CAD build for the part. Positions are in the model's coordinates, mm. Round coordinates to 2 decimals unless told otherwise and drop trailing zeros. Loops run counter-clockwise (first coordinate to the right, second up) from the corner with the lowest first, then second, coordinate; pieces in that order, holes last.
Autodesk Inventor part; units mm, degrees
ref_plane "YZ Plane" through (0, 0, 0) normal (1, 0, 0) x (0, 1, 0)
ref_plane "XZ Plane" through (0, 0, 0) normal (0, 1, 0) x (-1, 0, 0)
ref_plane "XY Plane" through (0, 0, 0) normal (0, 0, 1) x (1, 0, 0)
sketch "Sketch1" plane through (0, 0, 0) normal (0, 1, 0) x (-1, 0, 0)
  line L0 (0, 0) -> (-298.45, 0)
  line L1 (-298.45, 0) -> (-298.45, 171.45)
  line L2 (-298.45, 171.45) -> (0, 171.45)
  line L3 (0, 171.45) -> (0, 0)
  dimension "d0" = 298.45
  dimension "d1" = 171.45
extrude "Extrusion1" add sketch "Sketch1" along normal blind 6.35
sketch "Sketch3" plane through (0, 6.35, 0) normal (0, 1, 0) x (1, 0, 0)
  circle A0 centre (198.2183, -6.35) radius 3.3782
  circle A1 centre (100.2317, -6.35) radius 3.3782
  circle A2 centre (292.1, -57.8984) radius 3.3782
  circle A3 centre (292.1, -113.5516) radius 3.3782
  circle A4 centre (198.2183, -165.1) radius 3.3782
  circle A5 centre (100.2317, -165.1) radius 3.3782
  circle A6 centre (6.35, -57.8984) radius 3.3782
  circle A7 centre (6.35, -113.5516) radius 3.3782
  point P0 (0, 0)
extrude "Extrusion2" cut sketch "Sketch3" against normal up to next
fillet "Fillet1" radius 3.175 4 edges at (298.45, 3.175, 171.45) (0, 3.175, 171.45) (0, 3.175, 0) (298.45, 3.175, 0)
properties part number "Base" material "ABS Plastic"
Item 1: Cut at A-A, the plane x = 6.35. Give the cut face in (y, z), plus the area to 3 significant figures.
Answers follow:
outline: (0, 0) - (6.35, 0) - (6.35, 54.52) - (0, 54.52) - close; (0, 61.28) - (6.35, 61.28) - (6.35, 110.17) - (0, 110.17) - close; (0, 116.93) - (6.35, 116.93) - (6.35, 171.45) - (0, 171.45) - close
area: 1,000 mm2
Item 2: Two-plate mould, pull along Z, no slides. Class faces 1 (the flat face through (147, 3, 0)), 2 (the cylindrical face through (293.66, 3.22, 116.55)), 3 (the flat face through (151, 0, 87)): released by +Z, released by -Z, zero draft, split by the parting line, or undercut.
Answers follow:
face 1: released by -Z
face 2: undercut
face 3: zero draft
Item 3: Cut at B-B, the plane z = 6.35. Give the cut face in (x, y), plus the area to 3 significant figures.
Answers follow:
outline: (0, 0) - (96.85, 0) - (96.85, 6.35) - (0, 6.35) - close; (103.61, 0) - (194.84, 0) - (194.84, 6.35) - (103.61, 6.35) - close; (201.6, 0) - (298.45, 0) - (298.45, 6.35) - (201.6, 6.35) - close
area: 1,810 mm2
Item 4: Probe line 1 (X direction, y = 4.25, z = 115). List the from-to ranges inside material, lowest first.
Answers follow:
line 1: x = 0 to 3.3, 9.4 to 289.05, 295.15 to 298.45
